from build123d import *

# Parameters (mm, degrees)
SKETCH1_R           = 6
BOSS_EXTRUDE1_DEPTH = 2
BOSS_EXTRUDE2_DEPTH = 8
SKETCH3_R           = 5
BOSS_EXTRUDE3_DEPTH = 4
SKETCH4_R           = 2
CUT_EXTRUDE1_DEPTH  = 0.2
FILLET1_R           = 1


with BuildPart() as part:
    # Sketch1 → Boss-Extrude1 (new body)
    with BuildSketch(Plane(origin=(0, 0, 0), x_dir=(1, 0, 0), z_dir=(0, 1, 0))):
        with BuildLine():
            Line((1, 0), (39, 0))
            ThreePointArc((39, 0), (39.707106781, 0.292893219), (40, 1))
            Line((40, 1), (40, 19))
            ThreePointArc((40, 19), (39.707106781, 19.707106781), (39, 20))
            Line((39, 20), (1, 20))
            ThreePointArc((1, 20), (0.292893219, 19.707106781), (0, 19))
            Line((0, 19), (0, 1))
            ThreePointArc((0, 1), (0.292893219, 0.292893219), (1, 0))
        make_face()
        with Locations(Location((20, 10, 0), (0, 0, 270))):
            Circle(SKETCH1_R, mode=Mode.SUBTRACT)
    extrude(amount=BOSS_EXTRUDE1_DEPTH)

    # Sketch2 → Boss-Extrude2 (add)
    with BuildSketch(Plane(origin=(0, 0, 0), x_dir=(1, 0, 0), z_dir=(0, 1, 0))):
        with BuildLine():
            Line((2, 1), (38, 1))
            ThreePointArc((38, 1), (38.707106781, 1.292893219), (39, 2))
            Line((39, 2), (39, 18))
            ThreePointArc((39, 18), (38.707106781, 18.707106781), (38, 19))
            Line((38, 19), (2, 19))
            ThreePointArc((2, 19), (1.292893219, 18.707106781), (1, 18))
            Line((1, 18), (1, 2))
            ThreePointArc((1, 2), (1.292893219, 1.292893219), (2, 1))
        make_face()
    extrude(amount=-BOSS_EXTRUDE2_DEPTH)

    # Sketch3 → Boss-Extrude3 (add)
    with BuildSketch(Plane(origin=(0, 0, 0), x_dir=(1, 0, 0), z_dir=(0, 1, 0))):
        with Locations(Location((20, 10, 0), (0, 0, 270))):
            Circle(SKETCH3_R)
    extrude(amount=BOSS_EXTRUDE3_DEPTH)

    # Sketch4 → Cut-Extrude1 (cut)
    with BuildSketch(Plane(origin=(0, 2, 0), x_dir=(1, 0, 0), z_dir=(0, 1, 0))):
        with Locations(Location((30, 10, 0), (0, 0, 270))):
            Circle(SKETCH4_R)
    extrude(amount=-CUT_EXTRUDE1_DEPTH, mode=Mode.SUBTRACT)

    # Fillet1
    fillet1_edges = [part.edges().sort_by_distance(p)[0] for p in [
        (39.707106781, 2, -0.292893219),
        (40, 2, -10),
        (39.707106781, 2, -19.707106781),
        (20, 2, -20),
        (0.292893219, 2, -19.707106781),
        (0, 2, -10),
        (0.292893219, 2, -0.292893219),
        (20, 4, -15),
        (20, 2, 0),
    ]]
    fillet(fillet1_edges, radius=FILLET1_R)


solid = part.part
The listing builds one solid part. Answer for the finished solid, in the listing's coordinates (mm). A direction names the side the tool comes from. Give positions to 0.01 mm unless a question says otherwise; leave off trailing zeros. Order: outer loops, then holes, each group sorted by start corner. A loop starts at its lowest first (then second) coordinate and runs counter-clockwise, first axis right, second up. Notation, with made-up numbers: (-16.5, 36) -> (11.5, 36) arc R10 ccw to (11.5, 54) -> close; hole circle Ø10 at (-23, 89.25). An arc over 180 degrees is marked (long way). Put each result on its own line as item: value.
Item 1: For a pull along X with two mould halves and no side action, classify faces 4 (the face through (38.699, -3.944, -1.285)), 5 (the face through (15.564, 1.479, -7.693)), 6 (the face through (20, -4, -1)) as released by +X, released by -X, zero draft, split by the parting line, or undercut.
Established:
face 4: released by +X
face 5: undercut
face 6: zero draft
Item 2: A cutting plane is placed at B-B on x = 30. Give the vertices of the cut face in (y, z), plus the area to 3 significant figures.
Established:
outline: (-8, -19) -> (0, -19) -> (0, -20) -> (1, -20) arc R1 ccw to (2, -19) -> (2, -12) -> (1.8, -12) -> (1.8, -8) -> (2, -8) -> (2, -1) arc R1 ccw to (1, 0) -> (0, 0) -> (0, -1) -> (-8, -1) -> close
area: 183 mm^2
Item 3: Straight lines are drawn through the part: line 1 (X direction, y = 0.8, z = -10); line 2 (Y direction, x = 6.5, z = -16); line 3 (Z direction, x = 33, y = -3.5). For each, find the intervals that lie inside material, in ascending order.
Established:
line 1: x = 0 to 14, 15 to 25, 26 to 40
line 2: y = -8 to 2
line 3: z = -19 to -1
Item 4: A cutting plane is placed at A-A on z = -10. Give the vertices of the cut face in (x, y), plus the area to 3 significant figures.
Established:
outline: (0, 0) -> (1, 0) -> (1, -8) -> (39, -8) -> (39, 0) -> (40, 0) -> (40, 1) arc R1 ccw to (39, 2) -> (32, 2) -> (32, 1.8) -> (28, 1.8) -> (28, 2) -> (26, 2) -> (26, 0) -> (25, 0) -> (25, 3) arc R1 ccw to (24, 4) -> (16, 4) arc R1 ccw to (15, 3) -> (15, 0) -> (14, 0) -> (14, 2) -> (1, 2) arc R1 ccw to (0, 1) -> close
area: 398 mm^2
Item 5: A cutting plane is placed at D-D on x = 8.5. Give the vertices of the cut face in (y, z).
Established:
outline: (-8, -19) -> (0, -19) -> (0, -20) -> (1, -20) arc R1 ccw to (2, -19) -> (2, -1) arc R1 ccw to (1, 0) -> (0, 0) -> (0, -1) -> (-8, -1) -> close
Item 6: For faces 1 (the face through (1, -4, -10)), 2 (the face through (1.301, -3.944, -18.715)), 3 (the face through (18.4, 0, -0.4)), determine the directions among +Z, -Z, +X, -X, +Y, -Y from which every point of the face is accessible in a straight line to the end or side of a thin tool.
Established:
face 1: +Z, -Z, -X, -Y
face 2: -Z, -X, -Y
face 3: -Y
Item 7: Given P1, Ø1.5, axis at x = 13.5, y = -3, coming from the +Z side; P2, Ø6.5, axis at x = 13.5, y = -2.5, coming from the -Z side; P3, Ø2.5, axis at y = -2, z = -11, coming from the +X side; P4, Ø6.5, axis at y = -4, z = -7.5, coming from the -X side, each flat-ended and moving along its own axis, determine where each tip first touches the part or whether it passes through.
Established:
P1: stops at z = -1
P2: stops at z = -20
P3: stops at x = 39
P4: stops at x = 1
Item 8: A cutting plane is placed at C-C on y = -4. Give the vertices of the cut face in (x, z).
Established:
outline: (1, -18) arc R1 ccw to (2, -19) -> (38, -19) arc R1 ccw to (39, -18) -> (39, -2) arc R1 ccw to (38, -1) -> (2, -1) arc R1 ccw to (1, -2) -> close
